Design review of the part shown in the three views and the two pictorial views. Dimensions are in mm from the part's minimum x, y and z. A direction names the side the tool comes from. Coordinates: 2 decimals unless noted, no trailing zeros. Order: outer loops, then holes, each group sorted by start corner. A loop starts at its lowest first (then second) coordinate and runs counter-clockwise, first axis right, second up. Notation, with made-up numbers: (-21, 23) -> (-9, 23) arc R15 cw to (-9, 29) -> close; hole circle Ø4 at (-19.75, -15). An arc over 180 degrees is marked (long way). Answer as a JSON object with one key per item and string values. Group by question number.
1) Add section C-C, the plane y = 7.5. Write out the cut boundary in (x, z) (1 decimal).
2) Add section D-D, the plane y = 30.5. Write out the cut boundary in (x, z).
3) Machinability: for the marked faces 4, 5, 6 and 7, which of the approach directions +Z, -Z, +X, -X, +Y, -Y give a long, thin tool a straight path to every point of the face, cutting with its end or side? Answer none if there is none.
4) Add section B-B, the plane x = 34. Write out the cut boundary in (y, z) (1 decimal).
5) Wall thickness on L1, parallel to Y at x = 64.5, z = 44.5; L2, parallel to Z at x = 39.5, y = 19; L3, parallel to X at y = 24, z = 38.5 (1 decimal): over which ranges is each line inside the solid? List them lowest first.
6) For pin 1 (21.5 mm diameter, centred on x = 73, z = 33.5, fed in from +Y); pin 2 (10 mm diameter, centred on x = 30.5, y = 30, fed in from +Z); pin 3 (12 mm diameter, centred on x = 56.5, y = 46, fed in from +Z); pin 4 (2 mm diameter, centred on y = 22.5, z = 24.5, fed in from +X), all flat-tipped, find the tip position at first contact; note any pin that passes through.
7) Draft analysis for pull direction Y (two halves, no side actions). For the marked faces 1, 2 and 3, state which applies: +Y half, -Y half, draft (parallel to the pull), parting line (faces both ways), or undercut.
8) Add section A-A, the plane z = 25.5. Write out the cut boundary in (x, y) (1 decimal), then the cut area to 3 significant figures.
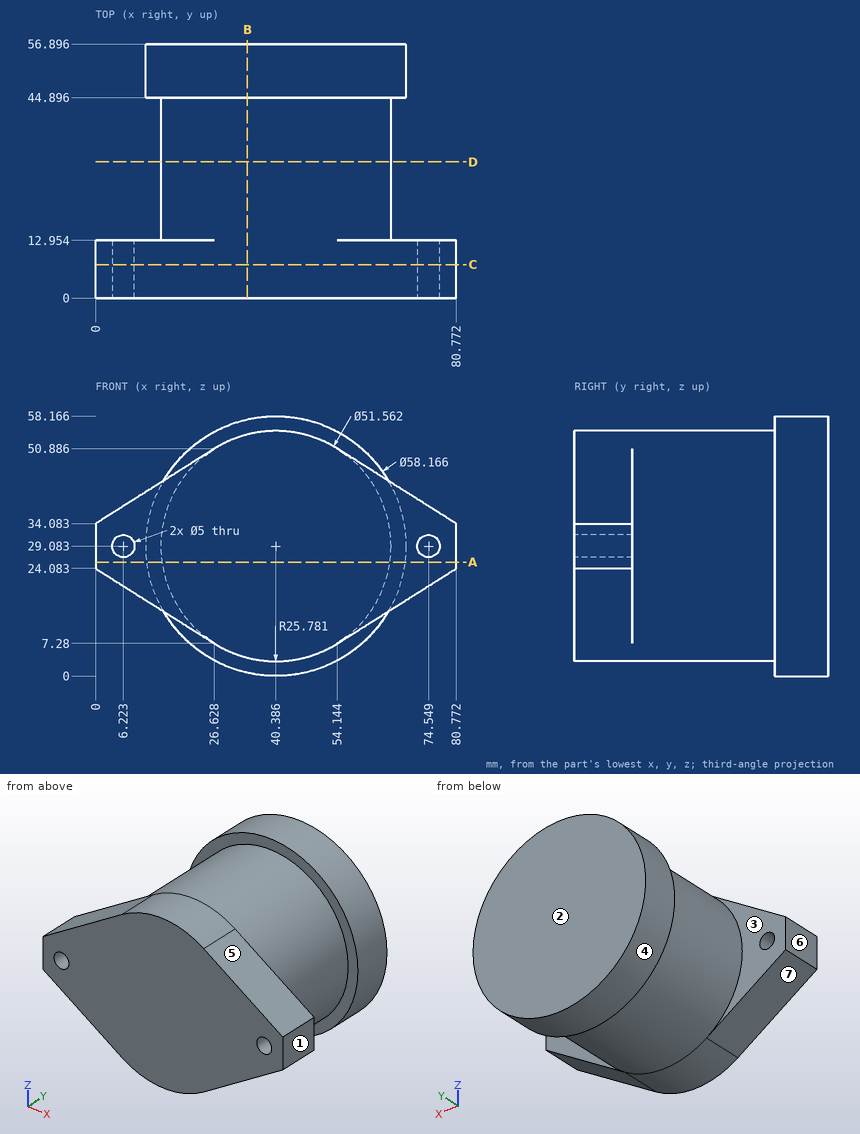
Output values:
{
 "1": {"outline": "(0, 24.1) -> (26.6, 7.3) arc R25.8 ccw to (54.1, 7.3) -> (80.8, 24.1) -> (80.8, 34.1) -> (54.1, 50.9) arc R25.8 ccw to (26.6, 50.9) -> (0, 34.1) -> close; hole circle Ø5 at (6.2, 29.1); hole circle Ø5 at (74.5, 29.1)"},
 "2": {"outline": "circle Ø51.56 at (40.39, 29.08)"},
 "3": {"face 4": "+Y", "face 5": "+Z, +X, -Y", "face 6": "+Z, -Z, -X, +Y, -Y", "face 7": "-Z, -X, -Y"},
 "4": {"outline": "(0, 4.1) -> (44.9, 4.1) -> (44.9, 0.7) -> (56.9, 0.7) -> (56.9, 57.5) -> (44.9, 57.5) -> (44.9, 54.1) -> (0, 54.1) -> close"},
 "5": {"L1": "y = 44.9 to 56.9", "L2": "z = 3.32 to 54.85", "L3": "x = 16.4 to 64.4"},
 "6": {"pin 1": "stops at y = 56.9", "pin 2": "stops at z = 54.4", "pin 3": "stops at z = 56.35", "pin 4": "stops at x = 65.92"},
 "7": {"face 1": "draft", "face 2": "+Y half", "face 3": "undercut"},
 "8": {"outline": "(0, 0) -> (80.8, 0) -> (80.8, 13) -> (65.9, 13) -> (65.9, 44.9) -> (69.2, 44.9) -> (69.2, 56.9) -> (11.5, 56.9) -> (11.5, 44.9) -> (14.9, 44.9) -> (14.9, 13) -> (0, 13) -> close", "area": "3,370 mm²"}
}
